Can you work these out from the model? Positions are in its coordinate system, mm. A direction names the side the tool comes from. Round coordinates to 2 decimals unless told otherwise and drop trailing zeros. Order: outer loops, then holes, each group sorted by start corner. A loop starts at its lowest first (then second) coordinate and runs counter-clockwise, first axis right, second up.
Q1. For faces 5 (the face through (-2.5, 6, -38)), 6 (the face through (0, 15, -29)), 7 (the face through (2.5, 6, -38)), which set-ups out of +Z, -Z, +X, -X, +Y, -Y let a thin tool reach every point of the face, with its end or its side?
Q2. If we section it at A-A (x = -0.75): Please give me the cut outline in (y, z), plus the area to 3 significant figures.
Q3. Will these pins go through, and if not, where does the flat tip stop? P1, Ø7, axis at x = 0, z = 9, coming from the +Y side; P2, Ø2, axis at y = 10, z = -46.5, coming from the -X side; P3, Ø2.5, axis at x = 0.5, y = 13.5, coming from the -Z side; P4, Ø4, axis at x = -0.5, z = -28.5, coming from the +Y side.
Q4. We'd pull the mould along Z, two halves only. Please class faces 1 (the face through (0, 2, -65.932)), 2 (the face through (6.126, 9.304, 11.088)), 3 (the face through (0, 13, 3)), 4 (the face through (9, 10, -6)): pulls with the +Z half, pulls with the -Z half, needs draft (parallel to the pull), parting line crosses it, or undercut.
Q5. If we section it at C-C (y = 4.25): Please give me the cut outline in (x, z), plus the area to 3 significant figures.
Q6. If we section it at B-B (z = 9): Please give me the cut outline in (x, y), plus the area to 3 significant figures.
Q7. If I drill on line 1 (X direction, y = 8.5, z = 9); line 2 (Z direction, x = 2.5, y = 18.75); line 3 (Z direction, x = 0, y = 6.75), over which ranges is the centre line in solid material (lowest first)?
from build123d import *

# Parameters (mm, degrees)
EXTRUDE_1_DEPTH     = 9
EXTRUDE_2_DEPTH     = 2.5
SKETCH_2_R          = 6
CUT_EXTRUDE_1_DEPTH = 35
FILLET_2_R          = 2


with BuildPart() as part:
    # Sketch 1 → Extrude 1 (new, symmetric)
    with BuildSketch(Plane(origin=(0, 0, 0), x_dir=(0, 0, -1), z_dir=(1, 0, 0))):
        Polygon((20.931942518, 0), (0, 0), (-19.068057482, 16), (-19.068057482, 20), (20.931942518, 20), align=None)
    extrude(amount=EXTRUDE_1_DEPTH, both=True)

    # Sketch 1_3 → Extrude 2 (add, symmetric)
    with BuildSketch(Plane(origin=(0, 0, 0), x_dir=(0, 0, -1), z_dir=(1, 0, 0))):
        Polygon((20.931942518, 15), (20.931942518, 0), (65.931942518, 0), (65.931942518, 5), (50.931942518, 5), (50.931942518, 10), (35.931942518, 10), (35.931942518, 15), align=None)
    extrude(amount=EXTRUDE_2_DEPTH, both=True)

    # Sketch 2 → Cut-Extrude 1 (cut)
    with BuildSketch(Plane(origin=(0, 20, 0), x_dir=(1, 0, 0), z_dir=(0, 1, 0))):
        with Locations(Location((0, -9, 0), (0, 0, 270))):
            Circle(SKETCH_2_R)
    extrude(amount=-CUT_EXTRUDE_1_DEPTH, mode=Mode.SUBTRACT)

    # Fillet 2
    fillet_2_edges = [part.edges().sort_by_distance(p)[0] for p in [
        (0, 16, 19.068057482),
        (0, 20, 19.068057482),
        (9, 18, 19.068057482),
        (-9, 18, 19.068057482),
    ]]
    fillet(fillet_2_edges, radius=FILLET_2_R)


solid = part.part
Solution:
1. face 5: -Z, -X, +Y, -Y
1. face 6: -Z, +X, -X, +Y
1. face 7: -Z, +X, +Y, -Y
2. outline: (0, -65.93) - (5, -65.93) - (5, -50.93) - (10, -50.93) - (10, -35.93) - (15, -35.93) - (15, -20.93) - (20, -20.93) - (20, 3.05) - (2.56, 3.05) - (0, 0) - close; (12.55, 14.95) - (20, 14.95) - (20, 17.07) arc R2 ccw to (18, 19.07) - (16.93, 19.07) arc R2 ccw to (15.4, 18.35) - close
2. area: 948 mm2
3. P1: passes through
3. P2: stops at x = -2.5
3. P3: stops at z = -35.93
3. P4: stops at y = 15
4. face 1: pulls with the -Z half
4. face 2: pulls with the +Z half
4. face 3: undercut
4. face 4: needs draft
5. outline: (-9, -20.93) - (-2.5, -20.93) - (-2.5, -65.93) - (2.5, -65.93) - (2.5, -20.93) - (9, -20.93) - (9, 5.06) - (4.53, 5.06) arc R6 cw to (-4.53, 5.06) - (-9, 5.06) - close
5. area: 680 mm2
6. outline: (-9, 7.55) - (-6, 7.55) - (-6, 20) - (-9, 20) - close; (6, 7.55) - (9, 7.55) - (9, 20) - (6, 20) - close
6. area: 74.7 mm2
7. line 1: x = -9 to -6, 6 to 9
7. line 2: z = -20.93 to 3.55, 14.45 to 18.92
7. line 3: z = -50.93 to 3
